```python
from build123d import *

# Parameters (mm, degrees)
F0_W      = 102
F0_H      = 102
F1_DEPTH  = 3
F2_R      = 5
F3_R      = 5
F4_W      = 92
F4_H      = 92
F5_DEPTH  = 28
F6_R      = 5
F7_R      = 5
F8_T      = -2.5
F9_DEPTH  = 3
F10_DEPTH = 0.5


# Not quite as in the source:
# - an extrude ends at something that could not be found from the text; its depth is read off the source's solid


with BuildPart() as f1:
    # F0 (on Top) → F1 (new body)
    with BuildSketch(Plane.XY):
        Rectangle(F0_W, F0_H)
    extrude(amount=F1_DEPTH)

    # F2
    f2_edges = [f1.edges().sort_by_distance(p)[0] for p in [
        (-51, -51, 1.5),
        (51, -51, 1.5),
        (51, 51, 1.5),
    ]]
    fillet(f2_edges, radius=F2_R)

    # F3
    f3_edges = [f1.edges().sort_by_distance(p)[0] for p in [
        (-51, 51, 1.5),
    ]]
    fillet(f3_edges, radius=F3_R)

    # F4 (on face) → F5 (join)
    with BuildSketch(Plane.XY.offset(3)):
        Rectangle(F4_W, F4_H)
    extrude(amount=F5_DEPTH)

    # F6
    f6_edges = [f1.edges().sort_by_distance(p)[0] for p in [
        (-46, -46, 17),
    ]]
    fillet(f6_edges, radius=F6_R)

    # F7
    f7_edges = [f1.edges().sort_by_distance(p)[0] for p in [
        (46, -46, 17),
        (46, 46, 17),
        (-46, 46, 17),
    ]]
    fillet(f7_edges, radius=F7_R)

    # F8
    f8_openings = [f1.faces().sort_by_distance(p)[0] for p in [
        (0, 0, 31),
    ]]
    offset(amount=F8_T, openings=f8_openings, kind=Kind.INTERSECTION)

    # F9 (add): faces of the model
    f9_faces = [f1.faces().sort_by_distance(p)[0] for p in [
        (-47.4424978336, 0, 3),
        (0, 0, 2.5),
    ]]
    extrude(f9_faces, amount=F9_DEPTH)

    # F10 (add, through all): a face of the model
    f10_faces = [f1.faces().sort_by_distance(p)[0] for p in [
        (0, 0, 5.5),
    ]]
    extrude(f10_faces, amount=F10_DEPTH)


solid = f1.part
```
Here's how the part is built. I have some questions about the finished solid (model axes, mm). A direction names the side the tool comes from. Round coordinates to 2 decimals unless told otherwise and drop trailing zeros. Order: outer loops, then holes, each group sorted by start corner. A loop starts at its lowest first (then second) coordinate and runs counter-clockwise, first axis right, second up. Notation, with made-up numbers: M 27,-32 L 60,-32 A22 cw 60,-18 Z; hole C 44,32 d8. An arc over 180 degrees is marked long. Answer in a Markdown table with one row per item.
Item 1: Imagine slicing it at A-A, the plane z = 10.5. Write out the boundary of the cut face in (x, y), and give its area (3 significant figures).
A:
| item | result |
|---|---|
| outline | M -46,-41 A5 ccw -41,-46 L 41,-46 A5 ccw 46,-41 L 46,41 A5 ccw 41,46 L -41,46 A5 ccw -46,41 Z; hole M -43.5,-41 A2.5 ccw -41,-43.5 L 41,-43.5 A2.5 ccw 43.5,-41 L 43.5,41 A2.5 ccw 41,43.5 L -41,43.5 A2.5 ccw -43.5,41 Z |
| area | 879 mm2 |
Item 2: I'm going to push flat-ended pins straight in: pin 1 (2 mm diameter, centred on x = 5.5, z = 26, fed in from -Y); pin 2 (5 mm diameter, centred on y = -30, z = 24, fed in from -X); pin 3 (4 mm diameter, centred on y = -15.5, z = 14, fed in from +X); pin 4 (3 mm diameter, centred on x = -4, z = 7, fed in from +Y). Where does each tip first touch, or does it pass through?
A:
| item | result |
|---|---|
| pin 1 | stops at y = -46 |
| pin 2 | stops at x = -46 |
| pin 3 | stops at x = 46 |
| pin 4 | stops at y = 51 |
Item 3: For faces 1 (the face through (44, -45, 19)), 2 (the face through (-46, -1, 18)), 3 (the face through (-45, 44, 19)), 4 (the face through (-42.748, -42.787, 18.675)), which set-ups out of +Z, -Z, +X, -X, +Y, -Y let a thin tool reach every point of the face, with its end or its side?
A:
| item | result |
|---|---|
| face 1 | +Z, +X, -Y |
| face 2 | +Z, -X, +Y, -Y |
| face 3 | +Z, -X, +Y |
| face 4 | +Z |
Item 4: Imagine slicing it at B-B, the plane x = -35.5. Write out the boundary of the cut face in (y, z), and give its area (3 significant figures).
A:
| item | result |
|---|---|
| outline | M -51,0 L 51,0 L 51,6 L 46,6 L 46,31 L 43.5,31 L 43.5,6 L -43.5,6 L -43.5,31 L -46,31 L -46,6 L -51,6 Z |
| area | 737 mm2 |
Item 5: If I drill on L1, parallel to X at y = 6, z = 6.5; L2, parallel to Z at x = 39, y = -8, over which ranges is the centre line in solid material (lowest first)? Write a range as from..to.
A:
| item | result |
|---|---|
| L1 | x = -46..-43.5, 43.5..46 |
| L2 | z = 0..6 |
Item 6: Thinking about a two-plate mould opening in Y: for faces 5 (the face through (45, 44, 19)), 6 (the face through (-1, -43.5, 18)), 7 (the face through (42.787, 42.748, 18.675)), 8 (the face through (-1, -46, 18)), which applies, +Y half, -Y half, draft (parallel to the pull), parting line (faces both ways), or undercut?
A:
| item | result |
|---|---|
| face 5 | +Y half |
| face 6 | undercut |
| face 7 | undercut |
| face 8 | -Y half |
